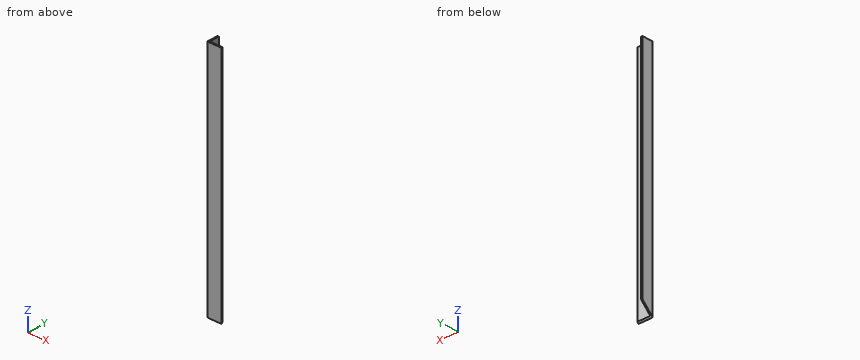
```python
from build123d import *

# Parameters (mm, degrees)
BOSS_EXTRUDE1_DEPTH = 360
CUT_EXTRUDE1_DEPTH  = 360


with BuildPart() as part:
    # Sketch2 → Boss-Extrude1 (new body)
    with BuildSketch(Plane.XY):
        Polygon((0, 0), (0, 17), (2, 17), (2, 2), (22, 2), (22, 0), align=None)
    extrude(amount=BOSS_EXTRUDE1_DEPTH)

    # Sketch3 → Cut-Extrude1 (cut)
    with BuildSketch(Plane.ZY):
        Polygon((0, 0), (17, 17), (0, 17), align=None)
    extrude(amount=-CUT_EXTRUDE1_DEPTH, mode=Mode.SUBTRACT)


solid = part.part
```
Read the model definition and answer for the solid it produces. Units are mm, in the model's axes. Coordinates: 2 decimals unless noted, no trailing zeros. Loops run counter-clockwise (first coordinate to the right, second up) from the corner with the lowest first, then second, coordinate; pieces in that order, holes last. Notation, with made-up numbers: (85, 36) -> (103, 36) arc R34 cw to (103, 69) -> close; hole circle Ø8 at (-20.5, 5.5). An arc over 180 degrees is marked (long way). Return JSON: item names as keys, results as strings.
Item 1: Flat-ended cylindrical pins translate along their axes: P1, Ø6, axis at y = 14.5, z = 170, coming from the +X side; P2, Ø12, axis at x = 14.5, z = 158, coming from the +Y side; P3, Ø12, axis at x = 5, z = 183.5, coming from the -Y side. Find the tip coordinate at first contact, or state that the pin passes through.
Answers:
{"P1": "stops at x = 2", "P2": "stops at y = 2", "P3": "stops at y = 0"}
Item 2: Find section C-C (x = 8.5). Determine the outline of the cut face in (y, z), plus the area to 3 significant figures.
Answers:
{"outline": "(0, 0) -> (2, 2) -> (2, 360) -> (0, 360) -> close", "area": "718 mm2"}
Item 3: Find section B-B (y = 6.5). Determine the outline of the cut face in (x, z).
Answers:
{"outline": "(0, 6.5) -> (2, 6.5) -> (2, 360) -> (0, 360) -> close"}
Item 4: Find section A-A (z = 327). Determine the outline of the cut face in (x, y).
Answers:
{"outline": "(0, 0) -> (22, 0) -> (22, 2) -> (2, 2) -> (2, 17) -> (0, 17) -> close"}
Item 5: Find the intervals of material crossed by probe 1 along X at (y, z) = (2.25, 18); probe 2 along Z at (x, y) = (1.5, 1.5), in increasing order.
Answers:
{"probe 1": "x = 0 to 2", "probe 2": "z = 1.5 to 360"}
